from build123d import *

# Parameters (mm, degrees)
F1_DEPTH  = 18
F4_W      = 390
F4_H      = 320
F5_DEPTH  = 18
F6_R      = 20
F8_DEPTH  = 25
F10_DEPTH = 18


with BuildPart() as f1:
    # F0 (on Front) → F1 (new body)
    with BuildSketch(Plane.XZ):
        Polygon((500, 1000), (18, 686.7), (18, 351), (782, 351), (782, 859), align=None)
    extrude(amount=F1_DEPTH)

    # F4 (on face) → F5 (cut, through all)
    with BuildSketch(Plane.XZ.offset(18)):
        with Locations((493, 561)):
            Rectangle(F4_W, F4_H)
    extrude(amount=-F5_DEPTH, mode=Mode.SUBTRACT)

    # F6
    f6_edges = [f1.edges().sort_by_distance(p)[0] for p in [
        (298, -9, 721),
        (688, -9, 721),
        (298, -9, 401),
        (688, -9, 401),
    ]]
    fillet(f6_edges, radius=F6_R)

    # F7 (on face) → F8 (cut)
    with BuildSketch(Plane.XZ.offset(18)):
        Polygon((458.077819, 972.750582), (416.155638, 945.501165), (425.965429, 930.40918), (467.887609, 957.658597), align=None)
    extrude(amount=-F8_DEPTH, mode=Mode.SUBTRACT)

    # F9 (on face) → F10 (cut, through all)
    with BuildSketch(Plane.XZ.offset(18)):
        Polygon((857.770876, 821.114562), (500, 1000), (491.950155, 983.900311), (849.721032, 805.014872), align=None)
    extrude(amount=-F10_DEPTH, mode=Mode.SUBTRACT)


solid = f1.part
The model under review builds one solid part; all positions refer to its coordinate system, in mm. A direction names the side the tool comes from. Give positions to 0.01 mm unless a question says otherwise; leave off trailing zeros. Loops run counter-clockwise (first coordinate to the right, second up) from the corner with the lowest first, then second, coordinate; pieces in that order, holes last. Notation, with made-up numbers: (14.25, -39) -> (46.25, -39) arc R20 ccw to (46.25, -35) -> close; hole circle Ø2 at (30.25, -10). An arc over 180 degrees is marked (long way). Answer as a JSON object with one key per item and string values. Group by question number.
Q1. Insertion check: pin 1 (6 mm diameter, centred on x = 475.5, y = -14, fed in from +Z) (3 decimals); pin 2 (4 mm diameter, centred on y = -14.5, z = 812, fed in from -X); pin 3 (2 mm diameter, centred on x = 98, y = -14, fed in from +Z). Each pin has a flat end and moves straight along its axis. Give the tip position at first contact, or say it passes through.
Q2. Draft analysis for pull direction X (two halves, no side actions). For faces 1 (the flat face through (395, -9, 351)), 2 (the cylindrical face through (682.297, -8.874, 714.986)), 3 (the flat face through (496, -9, 992)), state which applies: pulls with the +X half, pulls with the -X half, needs draft (parallel to the pull), parting line crosses it, or undercut.
Q3. Take a section at C-C (y = -12.5). Write out the cut boundary in (x, z).
Q4. Tool access review of faces 4 (the flat face through (446.63, -9.13, 943.84)), 5 (the flat face through (463.05, -9.13, 965.1)), 6 (the flat face through (420.992, -9.126, 938.061)): name each direction out of +Z, -Z, +X, -X, +Y, -Y from which nothing blocks a thin tool from reaching the whole face with its end or side.
Q5. Take a section at D-D (z = 753). Write out the cut boundary in (x, y), plus the area to 3 significant figures.
Q6. Take a section at A-A (z = 529). Write out the cut boundary in (x, y), plus the area to 3 significant figures.
Q7. Take a section at B-B (x = 349). Write out the cut boundary in (y, z), plus the area to 3 significant figures.
Q8. Wall thickness on line 1 along Z through (x, y) = (461, -8); line 2 along Z through (x, y) = (625, -2); line 3 along X through (y, z) = (-4, 711): over which ranges is each line inside the solid? List them lowest first.
Answer below:
{
 "1": {"pin 1": "stops at z = 986.025", "pin 2": "stops at x = 207.69", "pin 3": "stops at z = 739.35"},
 "2": {"face 1": "needs draft", "face 2": "undercut", "face 3": "pulls with the +X half"},
 "3": {"outline": "(18, 351) -> (782, 351) -> (782, 838.88) -> (491.95, 983.9) -> (500, 1000) -> (458.08, 972.75) -> (467.89, 957.66) -> (425.97, 930.41) -> (416.16, 945.5) -> (18, 686.7) -> close; hole (298, 421) arc R20 ccw to (318, 401) -> (668, 401) arc R20 ccw to (688, 421) -> (688, 701) arc R20 ccw to (668, 721) -> (318, 721) arc R20 ccw to (298, 701) -> close"},
 "4": {"face 4": "+Y, -Y", "face 5": "-X, +Y, -Y", "face 6": "+Z, +Y, -Y"},
 "5": {"outline": "(120, -18) -> (782, -18) -> (782, 0) -> (120, 0) -> close", "area": "11,900 mm2"},
 "6": {"outline": "(18, -18) -> (298, -18) -> (298, 0) -> (18, 0) -> close; (688, -18) -> (782, -18) -> (782, 0) -> (688, 0) -> close", "area": "6,730 mm2"},
 "7": {"outline": "(-18, 351) -> (0, 351) -> (0, 401) -> (-18, 401) -> close; (-18, 721) -> (0, 721) -> (0, 901.85) -> (-18, 901.85) -> close", "area": "4,160 mm2"},
 "8": {"line 1": "z = 351 to 401, 721 to 953.18, 968.25 to 974.65", "line 2": "z = 351 to 401, 721 to 917.38", "line 3": "x = 55.38 to 300.68, 685.32 to 782"}
}
